from build123d import *

# Parameters (mm, degrees)
F0_W     = 2233
F0_H     = 270
F0_W_2   = 2195
F0_H_2   = 232
F1_DEPTH = 862.5
F2_W     = 2083
F2_H     = 1575
F3_DEPTH = 38
F4_W     = 2157
F4_H     = 1649
F4_W_2   = 2119
F4_H_2   = 1611
F5_DEPTH = 50
F6_W     = 2033
F6_H     = 1525
F7_DEPTH = 25


with BuildPart() as f1:
    # F0 (on Front) → F1 (new body, symmetric)
    with BuildSketch(Plane.XZ):
        with Locations((1116.5, 135)):
            Rectangle(F0_W, F0_H)
        with Locations((1116.5, 135)):
            Rectangle(F0_W_2, F0_H_2, mode=Mode.SUBTRACT)
    extrude(amount=F1_DEPTH, both=True)

    # F2 (on face) → F3 (cut)
    with BuildSketch(Plane.XY.offset(270)):
        with Locations((1116.5, 0)):
            Rectangle(F2_W, F2_H)
    extrude(amount=-F3_DEPTH, mode=Mode.SUBTRACT)

    # F4 (on face) → F5 (join)
    with BuildSketch(Plane(origin=(0, 0, 0), x_dir=(1, 0, 0), z_dir=(0, 0, -1))):
        with Locations((1116.5, 0)):
            Rectangle(F4_W, F4_H)
        with Locations((1116.5, 0)):
            Rectangle(F4_W_2, F4_H_2, mode=Mode.SUBTRACT)
    extrude(amount=F5_DEPTH)

    # F6 (on face) → F7 (cut)
    with BuildSketch(Plane(origin=(0, 0, 0), x_dir=(1, 0, 0), z_dir=(0, 0, -1))):
        with Locations((1116.5, 0)):
            Rectangle(F6_W, F6_H)
    extrude(amount=-F7_DEPTH, mode=Mode.SUBTRACT)


solid = f1.part
Geometry check sheet. Reference: the model listing, model coordinates, mm. A direction names the side the tool comes from. Give positions to 0.01 mm unless a question says otherwise; leave off trailing zeros. Loops run counter-clockwise (first coordinate to the right, second up) from the corner with the lowest first, then second, coordinate; pieces in that order, holes last.
(1) Section check B-B on y = -234. Record the cut outline in (x, z).
From the geometry:
outline: (0, 0) - (38, 0) - (38, -50) - (57, -50) - (57, 0) - (100, 0) - (100, 19) - (19, 19) - (19, 251) - (75, 251) - (75, 270) - (0, 270) - close; (2133, 0) - (2176, 0) - (2176, -50) - (2195, -50) - (2195, 0) - (2233, 0) - (2233, 270) - (2158, 270) - (2158, 251) - (2214, 251) - (2214, 19) - (2133, 19) - close
(2) Section check C-C on x = 1819. Record the cut outline in (y, z).
From the geometry:
outline: (-862.5, 0) - (-824.5, 0) - (-824.5, -50) - (-805.5, -50) - (-805.5, 0) - (-762.5, 0) - (-762.5, 19) - (-862.5, 19) - close; (-862.5, 251) - (-787.5, 251) - (-787.5, 270) - (-862.5, 270) - close; (762.5, 0) - (805.5, 0) - (805.5, -50) - (824.5, -50) - (824.5, 0) - (862.5, 0) - (862.5, 19) - (762.5, 19) - close; (787.5, 251) - (862.5, 251) - (862.5, 270) - (787.5, 270) - close
(3) Release check for a two-part mould opening along X. For faces 5 (the flat face through (0, -12, 133)), 6 (the flat face through (1102, -805.5, -25)), 7 (the flat face through (2233, -12, 133)), 8 (the flat face through (1111, 862.5, 256)) record: released by +X, released by -X, zero draft, split by the parting line, or undercut.
From the geometry:
face 5: released by -X
face 6: undercut
face 7: released by +X
face 8: zero draft
(4) Depth check by flat-ended pin: pin 1 Ø15 at (x, z) = (1081, -18.5) entering from -Y; pin 2 Ø9.5 at (y, z) = (-77, 263) entering from -X; pin 3 Ø25 at (y, z) = (153, -31) entering from +X. Enter the tip coordinate at first touch or a pass-through.
From the geometry:
pin 1: stops at y = -824.5
pin 2: stops at x = 0
pin 3: stops at x = 2195
(5) Set-up check for faces 1 (the flat face through (2195, 12, -25)), 2 (the flat face through (2176, 11, -25)), 3 (the flat face through (2214, -12, 133)), 4 (the flat face through (38, 12, -25)): record each of +Z, -Z, +X, -X, +Y, -Y from which the full face is reachable in a straight line by a thin tool's end or side.
From the geometry:
face 1: -Z, +X, +Y, -Y
face 2: -Z
face 3: +Y, -Y
face 4: -Z, -X, +Y, -Y
(6) Section check A-A on z = 180. Record the cut outline in (x, y), then the cut area to 4 significant figures.
From the geometry:
outline: (0, -862.5) - (19, -862.5) - (19, 862.5) - (0, 862.5) - close; (2214, -862.5) - (2233, -862.5) - (2233, 862.5) - (2214, 862.5) - close
area: 65,550 mm2
(7) Thickness scan on L1, parallel to X at y = -415, z = 232; L2, parallel to X at y = 98.5, z = -33.5; L3, parallel to Y at x = 145, z = -11.5. Record the ranges inside material, lowest first.
From the geometry:
L1: x = 0 to 19, 2214 to 2233
L2: x = 38 to 57, 2176 to 2195
L3: y = -824.5 to -805.5, 805.5 to 824.5
